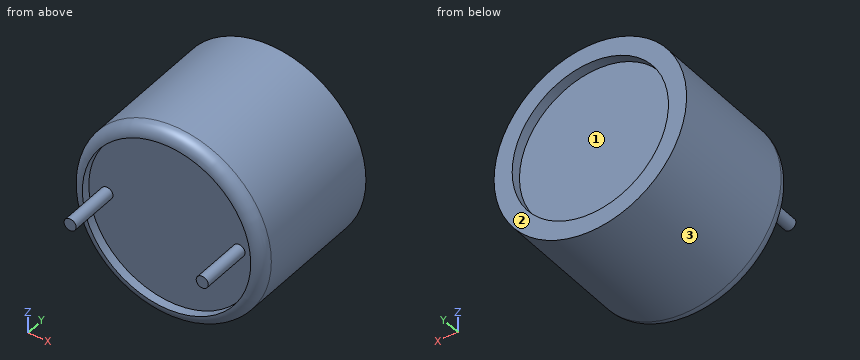
```python
from build123d import *

# Parameters (mm, degrees)
SKETCH1_R           = 7.975
BOSS_EXTRUDE1_DEPTH = 12.05
FILLET1_R           = 1
SKETCH3_R           = 6.975
CUT_EXTRUDE1_DEPTH  = 0.75
SKETCH4_R           = 0.5
BOSS_EXTRUDE2_DEPTH = 4.3
SKETCH5_R           = 6.475
CUT_EXTRUDE2_DEPTH  = 0.85


with BuildPart() as part:
    # Sketch1 → Boss-Extrude1 (new body)
    with BuildSketch(Plane(origin=(0, 0, 0), x_dir=(1, 0, 0), z_dir=(0, 1, 0))):
        Circle(SKETCH1_R)
    extrude(amount=BOSS_EXTRUDE1_DEPTH)

    # Fillet1
    fillet1_edges = [part.edges().sort_by_distance(p)[0] for p in [
        (-7.975, 0, 0),
    ]]
    fillet(fillet1_edges, radius=FILLET1_R)

    # Sketch3 → Cut-Extrude1 (cut)
    with BuildSketch(Plane.XZ):
        Circle(SKETCH3_R)
    extrude(amount=-CUT_EXTRUDE1_DEPTH, mode=Mode.SUBTRACT)

    # Sketch4 → Boss-Extrude2 (add)
    with BuildSketch(Plane.XZ.offset(-0.75)):
        with Locations((-5.475, 0)):
            Circle(SKETCH4_R)
        with Locations((5.475, 0)):
            Circle(SKETCH4_R)
    extrude(amount=BOSS_EXTRUDE2_DEPTH)

    # Sketch5 → Cut-Extrude2 (cut)
    with BuildSketch(Plane(origin=(0, 12.05, 0), x_dir=(1, 0, 0), z_dir=(0, 1, 0))):
        Circle(SKETCH5_R)
    extrude(amount=-CUT_EXTRUDE2_DEPTH, mode=Mode.SUBTRACT)


solid = part.part
```
Verification items for the finished model (mm, model axes). Face numbers are marked on the shaded views. Coordinates: 2 decimals unless noted, no trailing zeros. Write each loop counter-clockwise with the first axis right and the second up, starting at its lowest first coordinate (ties: lowest second). Pieces come first, ordered by that corner, then holes. Notation, with made-up numbers: M 15,10 L 29,10 A24 cw 29,33 Z; hole C 15.5,41.5 d9. An arc over 180 degrees is marked long. Answer as a JSON object with one key per item and string values. Group by question number.
(1) Cross-section at D-D, the plane y = 5.5. Record the cut outline in (x, z) (3 decimals).
(2) Gauge pin test, flat ends, axial feed: pin 1 (6 mm diameter, centred on y = 4.5, z = -4.5, fed in from +X); pin 2 (6 mm diameter, centred on x = 1.5, z = 0.5, fed in from -Y); pin 3 (5 mm diameter, centred on x = 4.5, y = 10.5, fed in from +Z). Record the tip position at first contact, or that the pin passes through.
(3) Material ranges on line 1 (Y direction, x = 4, z = 1.75); line 2 (X direction, y = 11.6, z = 0) (3 decimals); line 3 (Z direction, x = 0.25, y = 3.75), recorded low to high.
(4) Cross-section at A-A, the plane z = 0. Record the cut outline in (x, y) (3 decimals), and give its area (3 significant figures).
(5) Cross-section at C-C, the plane x = 0. Record the cut outline in (y, z) (3 decimals), and give its area (3 significant figures).
(6) Release check for a two-part mould opening along X. For the marked faces 1, 2 and 3 record: +X half, -X half, draft (parallel to the pull), parting line (faces both ways), or undercut.
(7) Cross-section at B-B, the plane y = -0.75. Record the cut outline in (x, z) (3 decimals), and give its area (3 significant figures).
Reply:
{
 "1": {"outline": "C 0,0 d15.95"},
 "2": {"pin 1": "x = 7.83", "pin 2": "y = 0.75", "pin 3": "z = 7.72"},
 "3": {"line 1": "0.75 to 11.2", "line 2": "-7.975 to -6.475, 6.475 to 7.975", "line 3": "-7.97 to 7.97"},
 "4": {"outline": "M -7.975,1 A1 ccw -6.975,0 L -6.975,0.75 L -5.975,0.75 L -5.975,-3.55 L -4.975,-3.55 L -4.975,0.75 L 4.975,0.75 L 4.975,-3.55 L 5.975,-3.55 L 5.975,0.75 L 6.975,0.75 L 6.975,0 A1 ccw 7.975,1 L 7.975,12.05 L 6.475,12.05 L 6.475,11.2 L -6.475,11.2 L -6.475,12.05 L -7.975,12.05 Z", "area": "179 mm²"},
 "5": {"outline": "M 0,-6.975 A1 ccw 1,-7.975 L 12.05,-7.975 L 12.05,-6.475 L 11.2,-6.475 L 11.2,6.475 L 12.05,6.475 L 12.05,7.975 L 1,7.975 A1 ccw 0,6.975 L 0.75,6.975 L 0.75,-6.975 Z", "area": "170 mm²"},
 "6": {"face 1": "undercut", "face 2": "draft", "face 3": "parting line"},
 "7": {"outline": "C -5.475,0 d1; C 5.475,0 d1", "area": "1.57 mm²"}
}
